The model under review builds one solid part; all positions refer to its coordinate system, in mm. Coordinates: 2 decimals unless noted, no trailing zeros. Write each loop counter-clockwise with the first axis right and the second up, starting at its lowest first coordinate (ties: lowest second). Pieces come first, ordered by that corner, then holes. Notation, with made-up numbers: (13.5, 49) - (53.5, 49) arc R7 ccw to (53.5, 59) - close; hole circle Ø2 at (54.5, 44.25). An arc over 180 degrees is marked (long way). Put each result on its own line as item: value.
from build123d import *

# Parameters (mm, degrees)
ESBO_O1_R                = 30
RESSALTO_EXTRUS_O1_DEPTH = 30
CORTE_EXTRUS_O1_DEPTH    = 30
CORTE_EXTRUS_O2_DEPTH    = 31


with BuildPart() as part:
    # Esboço1 → Ressalto-extrusão1 (new body)
    with BuildSketch(Plane(origin=(0, 0, 0), x_dir=(1, 0, 0), z_dir=(0, 1, 0))):
        Circle(ESBO_O1_R)
    extrude(amount=RESSALTO_EXTRUS_O1_DEPTH)

    # Esboço2 → Corte-extrusão1 (cut)
    with BuildSketch(Plane(origin=(0, 30, 0), x_dir=(1, 0, 0), z_dir=(0, 1, 0))):
        with BuildLine():
            Line((0, 30), (0, 0))
            Line((0, 0), (30, 0))
            ThreePointArc((30, 0), (-21.213203436, -21.213203436), (0, 30))
        make_face()
    extrude(amount=-CORTE_EXTRUS_O1_DEPTH, mode=Mode.SUBTRACT)

    # Esboço3 → Corte-extrusão2 (cut, through all)
    with BuildSketch(Plane.XY):
        Polygon((30, 30), (0, 12.679491924), (0, 30), align=None)
    extrude(amount=-CORTE_EXTRUS_O2_DEPTH, mode=Mode.SUBTRACT)


solid = part.part
1. To check wall thickness, follow probe 1 along Z at (x, y) = (11.5, 8.25); probe 2 along Y at (x, z) = (18.25, -7); probe 3 along Y at (x, z) = (13.25, -21.5). State the ranges of each line that lie inside material, in increasing order.
Determined:
probe 1: z = -27.71 to 0
probe 2: y = 0 to 23.22
probe 3: y = 0 to 20.33
2. For pin 1 Ø3 at (x, y) = (25.5, 15.5) entering from -Z; pin 2 Ø1.5 at (y, z) = (24, -21) entering from +X; pin 3 Ø6 at (x, z) = (12, -25.5) entering from +Y, all flat-tipped, find the tip position at first contact; note any pin that passes through.
Determined:
pin 1: stops at z = -18
pin 2: stops at x = 22.13
pin 3: stops at y = 21.34
3. Consider section D-D on y = 25.5. State the section outline as (x, z) points.
Determined:
outline: (22.21, -20.17) arc R30 ccw to (30, 0) - (22.21, 0) - close
4. Consider section C-C on x = 12. State the section outline as (y, z) points, plus the area to 3 significant figures.
Determined:
outline: (0, -27.5) - (19.61, -27.5) - (19.61, 0) - (0, 0) - close
area: 539 mm^2
5. Consider section A-A on y = 11.5. State the section outline as (x, z) points, plus the area to 3 significant figures.
Determined:
outline: (0, -30) arc R30 ccw to (30, 0) - (0, 0) - close
area: 707 mm^2
6. Consider section B-B on z = -27.5. State the section outline as (x, y) points.
Determined:
outline: (0, 0) - (11.99, 0) - (11.99, 19.6) - (0, 12.68) - close
